from build123d import *

# Parameters (mm, degrees)
SKETCH1_W           = 50
SKETCH1_H           = 80
BOSS_EXTRUDE1_DEPTH = 80
SKETCH4_W           = 50
SKETCH4_H           = 15
CUT_EXTRUDE2_DEPTH  = 124.693168769
FILLET1_R           = 50
SKETCH5_R           = 5
CUT_EXTRUDE3_DEPTH  = 25


with BuildPart() as part:
    # Sketch1 → Boss-Extrude1 (new body)
    with BuildSketch(Plane(origin=(0, 0, 0), x_dir=(0, 0, -1), z_dir=(1, 0, 0))):
        with Locations((25, 40)):
            Rectangle(SKETCH1_W, SKETCH1_H)
    extrude(amount=BOSS_EXTRUDE1_DEPTH)

    # Sketch4 → Cut-Extrude2 (cut, through all)
    with BuildSketch(Plane.XY):
        with Locations((40, 7.5)):
            Rectangle(SKETCH4_W, SKETCH4_H)
    extrude(amount=-CUT_EXTRUDE2_DEPTH, mode=Mode.SUBTRACT)

    # Fillet1
    fillet1_edges = [part.edges().sort_by_distance(p)[0] for p in [
        (40, 80, -50),
    ]]
    fillet(fillet1_edges, radius=FILLET1_R - 0.0001)  # a hair under: the kernel refuses the full size

    # Sketch5 → Cut-Extrude3 (cut)
    with BuildSketch(Plane.XZ.offset(-15)):
        with Locations(Location((40, -25, 0), (0, 0, 270))):
            Circle(SKETCH5_R)
    extrude(amount=-CUT_EXTRUDE3_DEPTH, mode=Mode.SUBTRACT)


solid = part.part
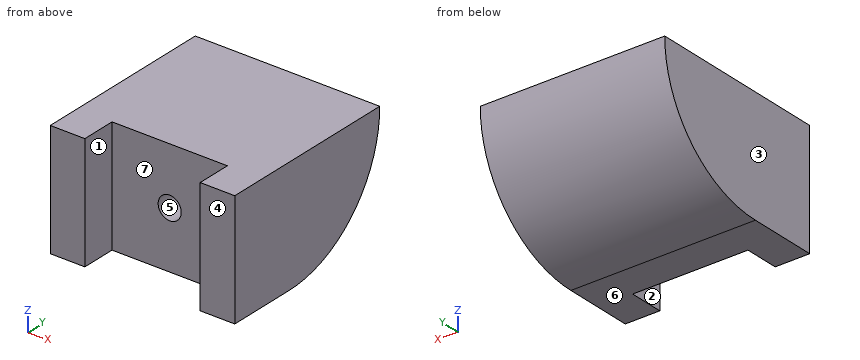
Source: CAD feature listing. Evaluate the final solid. Frame: model axes, mm. Face numbers are marked on the shaded views. A direction names the side the tool comes from. Round coordinates to 2 decimals unless told otherwise and drop trailing zeros. Write each loop counter-clockwise with the first axis right and the second up, starting at its lowest first coordinate (ties: lowest second). Pieces come first, ordered by that corner, then holes. Notation, with made-up numbers: M 33,22.25 L 60,22.25 A24 ccw 60,40.25 Z; hole C 82.5,63.5 d1. An arc over 180 degrees is marked long. One line per item, written item: value. Start each with the question number.
Item 1: Section query C-C (y = 23). Return the cut outline in (x, z).
Item 2: Ray query, L1, parallel to X at y = 9.5, z = -25; L2, parallel to X at y = 32, z = -25; L3, parallel to Z at x = 77, y = 70. Return the intervals inside material, ascending. Write a range as from..to.
Item 3: Pin query (flat end, axial travel): pin 1 (8 mm diameter, centred on x = 65.5, z = -43, fed in from +Y); pin 2 (10 mm diameter, centred on x = 46.5, z = -21, fed in from +Y); pin 3 (8 mm diameter, centred on x = 50.5, z = -25, fed in from -Y). Return the tip coordinate at first contact, or that it passes through.
Item 4: Section query A-A (y = 13.5). Return the cut outline in (x, z), plus the area to 3 significant figures.
Item 5: Section query D-D (z = -27). Return the cut outline in (x, y).
Item 6: Mould query, pull axis X, two halves, no side actions, for the marked faces 1, 2, 3 and 4. Classes: pulls with the +X half, pulls with the -X half, needs draft (parallel to the pull), parting line crosses it, or undercut.
Item 7: Set-up query: the marked faces 5, 6 and 7. Return all of +Z, -Z, +X, -X, +Y, -Y with unobstructed straight access to the full face (end or side cutting, diameter ignored); none if empty.
Result set:
1. outline: M 0,-50 L 80,-50 L 80,0 L 0,0 Z; hole C 40,-25 d10
2. L1: x = 0..15, 65..80
2. L2: x = 0..35, 45..80
2. L3: z = -30..0
3. pin 1: stops at y = 61.29
3. pin 2: stops at y = 77.37
3. pin 3: stops at y = 15
4. outline: M 0,-50 L 15,-50 L 15,0 L 0,0 Z; M 65,-50 L 80,-50 L 80,0 L 65,0 Z
4. area: 1,500 mm²
5. outline: M 0,0 L 15,0 L 15,15 L 35.42,15 L 35.42,40 L 44.58,40 L 44.58,15 L 65,15 L 65,0 L 80,0 L 80,72.08 L 0,72.08 Z
6. face 1: undercut
6. face 2: undercut
6. face 3: pulls with the -X half
6. face 4: needs draft
7. face 5: -Y
7. face 6: -Z, +X, -X, +Y, -Y
7. face 7: +Z, -Z, -Y
